The listing builds one solid part. Answer for the finished solid, in the listing's coordinates (mm). A direction names the side the tool comes from. Round coordinates to 2 decimals unless told otherwise and drop trailing zeros. Order: outer loops, then holes, each group sorted by start corner. A loop starts at its lowest first (then second) coordinate and runs counter-clockwise, first axis right, second up. Notation, with made-up numbers: M 52.5,10.5 L 61.5,10.5 A25 ccw 61.5,42.5 Z; hole C -8.5,-0.75 d10. An arc over 180 degrees is marked long. Write item = value, one per line. Start each with the question number.
(1) A cutting plane is placed at B-B, the plane y = 18. Determine the outline of the cut face in (x, z), and give its area (3 significant figures).
(2) Straight lines are drawn through the part: probe 1 along X at (y, z) = (17.5, -4.75); probe 2 along Y at (x, z) = (-8, 9.75) (3 decimals); probe 3 along Y at (x, z) = (-3, 2.5). For each, find the intervals that lie inside material, in ascending order. Write a range as from..to.
(3) For a pull along Z with two mould halves and no side action, classify faces 4 (the face through (7.7, 1.6, 10.1)), 5 (the face through (0, 0, 0)), 6 (the face through (-0.111, 43.54, 0.317)) as released by +Z, released by -Z, zero draft, split by the parting line, or undercut.
(4) A cutting plane is placed at A-A, the plane y = 40. Determine the outline of the cut face in (x, z), and give its area (3 significant figures).
(5) Each of these flat-tipped pins is pushed along its axis until it touches: pin 1 (1.5 mm diameter, centred on y = 43.5, z = -8, fed in from -X); pin 2 (1 mm diameter, centred on y = 9.5, z = 0.5, fed in from +X); pin 3 (1 mm diameter, centred on y = 35, z = -0.5, fed in from +X) (3 decimals); pin 4 (12.5 mm diameter, centred on x = -3, z = 2.5, fed in from +Y). Where does it stop, or does it pass through?
(6) Which of the six approach directions +Z, -Z, +X, -X, +Y, -Y give full straight-line access (tool end or side, diameter ignored) to faces 1 (the face through (4.6, 3.175, -11.2)), 2 (the face through (0.106, 45.243, 3.706)), 3 (the face through (0, 49, 3.429))?
from build123d import *

# Parameters (mm, degrees)
SKETCH4_2_W        = 17.78
SKETCH4_2_H        = 2.54
CUT_EXTRUDE4_DEPTH = 10.795
FILLET1_R          = 0.635


with BuildPart() as part:
    # Sketch1 → Revolve1 (revolve)
    with BuildSketch(Plane.XY, mode=Mode.PRIVATE) as revolve1_sk:
        with BuildLine():
            Line((0, 0), (12.7, 0))
            Line((12.7, 0), (12.7, 3.175))
            Line((12.7, 3.175), (11.938, 3.175))
            ThreePointArc((11.938, 3.175), (11.324664102, 7.361873807), (10.16, 11.43))
            ThreePointArc((10.16, 11.43), (11.43, 12.7), (10.16, 13.97))
            ThreePointArc((10.16, 13.97), (7.508321203, 25.917103348), (6.35, 38.1))
            ThreePointArc((6.35, 38.1), (7.576014134, 45.230603901), (2.507277216, 50.3936))
            ThreePointArc((2.507277216, 50.3936), (1.934406369, 52.446108137), (0, 53.34))
            Line((0, 53.34), (0, 50.8))
            Line((0, 50.8), (0, 0))
        make_face()
    revolve(revolve1_sk.sketch.rotate(Axis((0, 0, 0), (0, 1, 0)), 90), axis=Axis((0, 0, 0), (0, 1, 0)))

    # Sketch4 → Cut-Loft1 section 0
    with BuildSketch(Plane(origin=(0, 48.26, 0), x_dir=(1, 0, 0), z_dir=(0, 1, 0))):
        with BuildLine():
            Line((-8.89, -3.429), (8.89, -3.429))
            Line((8.89, -3.429), (8.89, -5.969))
            Line((8.89, -5.969), (-8.89, -5.969))
            Line((-8.89, -5.969), (-8.89, -3.429))
        make_face()
    # Sketch6 → Cut-Loft1 section 1
    with BuildSketch(Plane(origin=(0, 43.18, 0), x_dir=(1, 0, 0), z_dir=(0, 1, 0))):
        with BuildLine():
            Line((-8.89, -2.159), (8.89, -2.159))
            Line((8.89, -2.159), (8.89, 0.381))
            Line((8.89, 0.381), (-8.89, 0.381))
            Line((-8.89, 0.381), (-8.89, -2.159))
        make_face()
    loft(mode=Mode.SUBTRACT)

    # Sketch4<2> → Cut-Extrude4 (cut)
    with BuildSketch(Plane(origin=(0, 48.26, 0), x_dir=(1, 0, 0), z_dir=(0, 1, 0))):
        with Locations((0, -4.699)):
            Rectangle(SKETCH4_2_W, SKETCH4_2_H)
    extrude(amount=CUT_EXTRUDE4_DEPTH, mode=Mode.SUBTRACT)

    # Fillet1
    fillet1_edges = [part.edges().sort_by_distance(p)[0] for p in [
        (0, 43.18, 2.159),
        (0, 48.26, 3.429),
        (0, 43.18, -0.381),
    ]]
    fillet(fillet1_edges, radius=FILLET1_R)


solid = part.part
Reported:
q1.outline = C 0,0 d18.18
q1.area = 260 mm²
q2.probe_1 = -7.9..7.9
q2.probe_2 = 0..3.175
q2.probe_3 = 0..43.63, 47.02..49.77
q3.face_4 = split by the parting line
q3.face_5 = zero draft
q3.face_6 = undercut
q4.outline = C 0,0 d14.81
q4.area = 172 mm²
q5.pin_1 = -3.17
q5.pin_2 = 10.92
q5.pin_3 = 6.525
q5.pin_4 = 53.34
q6.face_1 = +Y
q6.face_2 = +X, -X
q6.face_3 = +Z, +X, -X, +Y
